```python
from build123d import *

# Parameters (mm, degrees)
F1_DEPTH  = 38.1
F2_T      = -3.175
F3_DEPTH  = 3.175
F4_W      = 3.175
F4_H      = 23.8125
F4_W_2    = 23.8125
F4_H_2    = 3.175
F5_DEPTH  = 7.9375
F6_W      = 55.5625
F6_H      = 55.5625
F6_R      = 2.15265
F6_W_2    = 31.75
F6_H_2    = 31.75
F7_DEPTH  = 3.175
F8_W      = 31.75
F8_H      = 31.75
F8_W_2    = 28.575
F8_H_2    = 28.575
F9_DEPTH  = 1.5875
F10_R     = 0.79375
F11_DEPTH = 7.9375
F12_W     = 1.5875
F12_H     = 31.75
F14_W     = 1.5875
F14_H     = 31.75


with BuildPart() as f1:
    # F0 (on Top) → F1 (new body)
    with BuildSketch(Plane.XY):
        with BuildLine():
            ThreePointArc((44.45, -44.45), (31.4308964237, -13.0191035763), (0, 0))
            Line((0, 0), (-9.525, 0))
            Line((-9.525, 0), (-9.525, -38.1))
            Line((-9.525, -38.1), (0, -38.1))
            ThreePointArc((0, -38.1), (4.4901280605, -39.9598719395), (6.35, -44.45))
            Line((6.35, -44.45), (6.35, -53.975))
            Line((6.35, -53.975), (44.45, -53.975))
            Line((44.45, -53.975), (44.45, -44.45))
        make_face()
    extrude(amount=F1_DEPTH)

    # F2
    f2_openings = [f1.faces().sort_by_distance(p)[0] for p in [
        (-9.525, -19.05, 19.05),
    ]]
    offset(amount=F2_T, openings=f2_openings)

    # F3 (cut, through all): a face of the model
    f3_faces = [f1.faces().sort_by_distance(p)[0] for p in [
        (25.4, -50.8, 19.05),
    ]]
    extrude(f3_faces, amount=-F3_DEPTH, mode=Mode.SUBTRACT)

    # F4 (on face) → F5 (cut)
    with BuildSketch(Plane(origin=(-9.525, 0, 0), x_dir=(0, -1, 0), z_dir=(-1, 0, 0))):
        with Locations((1.5875, 19.05)):
            Rectangle(F4_W, F4_H)
        with Locations((19.05, 36.5125)):
            Rectangle(F4_W_2, F4_H_2)
        with Locations((36.5125, 19.05)):
            Rectangle(F4_W, F4_H)
        with Locations((19.05, 1.5875)):
            Rectangle(F4_W_2, F4_H_2)
    extrude(amount=-F5_DEPTH, mode=Mode.SUBTRACT)

    # F6 (on face) → F7 (join)
    with BuildSketch(Plane.XZ.offset(53.975)):
        with Locations((25.4, 19.05)):
            Rectangle(F6_W, F6_H)
        with Locations((2.38125, -3.96875)):
            Circle(F6_R, mode=Mode.SUBTRACT)
        with Locations((48.41875, -3.96875)):
            Circle(F6_R, mode=Mode.SUBTRACT)
        with Locations((2.38125, 42.06875)):
            Circle(F6_R, mode=Mode.SUBTRACT)
        with Locations((25.4, 19.05)):
            Rectangle(F6_W_2, F6_H_2, mode=Mode.SUBTRACT)
        with Locations((48.41875, 42.06875)):
            Circle(F6_R, mode=Mode.SUBTRACT)
    extrude(amount=-F7_DEPTH)

    # F8 (on face) → F9 (join)
    with BuildSketch(Plane(origin=(-1.5875, 0, 0), x_dir=(0, -1, 0), z_dir=(-1, 0, 0))):
        with Locations((19.05, 19.05)):
            Rectangle(F8_W, F8_H)
        with Locations((19.05, 19.05)):
            Rectangle(F8_W_2, F8_H_2, mode=Mode.SUBTRACT)
    extrude(amount=-F9_DEPTH)

    # F10 (on face) → F11 (cut, through all)
    with BuildSketch(Plane(origin=(-1.5875, 0, 0), x_dir=(0, -1, 0), z_dir=(-1, 0, 0))):
        with Locations((3.175, 34.925)):
            Circle(F10_R)
        with Locations((3.175, 3.175)):
            Circle(F10_R)
        with Locations((34.925, 34.925)):
            Circle(F10_R)
        with Locations((34.925, 3.175)):
            Circle(F10_R)
    extrude(amount=F11_DEPTH, mode=Mode.SUBTRACT)

    # F13: sweep along a path in F13_path
    with BuildLine(Plane(origin=(9.525, -53.975, 34.925), x_dir=(0, -1, 0), z_dir=(0, 0, -1))) as f13_path:
        Line((0, 0), (-9.525, 0))
        ThreePointArc((-9.525, 0), (-16.2601920908, 2.7898079092), (-19.05, 9.525))
    # F12 (on face) → F13 (sweep)
    with BuildSketch(Plane.XZ.offset(53.975)):
        with Locations((10.31875, 19.05)):
            Rectangle(F12_W, F12_H)
    sweep(path=f13_path.line)

    # F15: sweep along a path in F15_path
    with BuildLine(Plane(origin=(41.275, -53.975, 34.925), x_dir=(0, -1, 0), z_dir=(0, 0, -1))) as f15_path:
        Line((0, 0), (-9.525, 0))
        ThreePointArc((-9.525, 0), (-38.7108323935, 12.0891676065), (-50.8, 41.275))
    # F14 (on face) → F15 (sweep)
    with BuildSketch(Plane.XZ.offset(53.975)):
        with Locations((40.48125, 19.05)):
            Rectangle(F14_W, F14_H)
    sweep(path=f15_path.line)


solid = f1.part
```
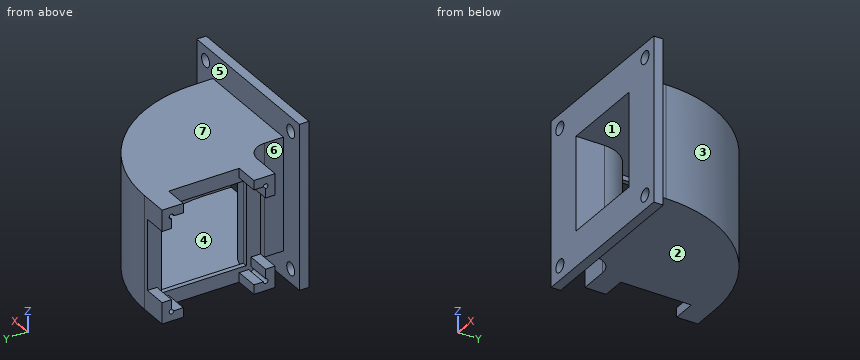
Verification items for the finished model (mm, model axes). Face numbers are marked on the shaded views. A direction names the side the tool comes from. Round coordinates to 2 decimals unless told otherwise and drop trailing zeros. Write each loop counter-clockwise with the first axis right and the second up, starting at its lowest first coordinate (ties: lowest second). Pieces come first, ordered by that corner, then holes.
1. Gauge pin test, flat ends, axial feed: P1, Ø3, axis at x = 8.5, z = 7, coming from the +Y side; P2, Ø1, axis at y = -10.5, z = 18.5, coming from the +X side; P3, Ø12, axis at x = 1.5, y = -9, coming from the +Z side. Record the tip position at first contact, or that the pin passes through.
2. Section check D-D on x = 48. Enter the section's corners in (y, z) (3 decimals).
3. Section check B-B on x = -4. Enter the section's corners in (y, z) (1 decimal).
4. Access from +Z, -Z, +X, -X, +Y, -Y to the whole of each face (thin tool, end or side, straight path). Record for the marked faces 5, 6 and 7.
5. Scan lines: L1, parallel to Z at x = 8, y = -15.5 (3 decimals); L2, parallel to Z at x = 15, y = -51 (3 decimals); L3, parallel to X at y = -50.5, z = 9.5. Record each from-to range of solid material in increasing order.
6. Draft check along X on the marked faces 1, 2, 3 and 4. Enter one of: +X half, -X half, draft (parallel to the pull), parting line (faces both ways), or undercut.
Answer:
1. P1: stops at y = -0.55
1. P2: stops at x = 29.27
1. P3: stops at z = 38.1
2. outline: (-53.975, -8.731) - (-50.8, -8.731) - (-50.8, -6.08) - (-53.975, -6.08) - close; (-53.975, -1.857) - (-50.8, -1.857) - (-50.8, 39.957) - (-53.975, 39.957) - close; (-53.975, 44.18) - (-50.8, 44.18) - (-50.8, 46.831) - (-53.975, 46.831) - close
3. outline: (-38.1, 0) - (-31, 0) - (-31, 3.2) - (-34.1, 3.2) arc R0.8 cw (long way) to (-34.9, 4) - (-34.9, 7.1) - (-38.1, 7.1) - close; (-38.1, 31) - (-34.9, 31) - (-34.9, 34.1) arc R0.8 cw (long way) to (-34.1, 34.9) - (-31, 34.9) - (-31, 38.1) - (-38.1, 38.1) - close; (-7.1, 0) - (0, 0) - (0, 7.1) - (-3.2, 7.1) - (-3.2, 4) arc R0.8 cw (long way) to (-4, 3.2) - (-7.1, 3.2) - close; (-7.1, 34.9) - (-4, 34.9) arc R0.8 cw (long way) to (-3.2, 34.1) - (-3.2, 31) - (0, 31) - (0, 38.1) - (-7.1, 38.1) - close
4. face 5: none
4. face 6: +Z, -Z, -X
4. face 7: +Z, +X, -X, +Y
5. L1: z = 0 to 3.175, 34.925 to 38.1
5. L2: z = -8.731 to 3.175, 34.925 to 46.831
5. L3: x = 6.35 to 11.11, 39.69 to 44.45
6. face 1: undercut
6. face 2: draft
6. face 3: +X half
6. face 4: undercut
